from build123d import *

# Parameters (mm, degrees)
F1_DEPTH = 6
F3_DEPTH = 3
F5_DEPTH = 9
F7_DEPTH = 3
F8_R     = 2
F9_R     = 2


with BuildPart() as f1:
    # F0 (on Top) → F1 (new body)
    with BuildSketch(Plane.XY):
        with BuildLine():
            Line((-3, 34.2), (-3, 0))
            ThreePointArc((-3, 0), (-2.1213203436, -2.1213203436), (0, -3))
            Line((0, -3), (34.2, -3))
            Line((34.2, -3), (34.2, 3))
            Line((34.2, 3), (5, 3))
            ThreePointArc((5, 3), (3.5857864376, 3.5857864376), (3, 5))
            Line((3, 5), (3, 34.2))
            Line((3, 34.2), (-3, 34.2))
        make_face()
        with BuildLine():
            Line((1, 32.2), (1, 2))
            ThreePointArc((1, 2), (1.2928932188, 1.2928932188), (2, 1))
            Line((2, 1), (32.2, 1))
            Line((32.2, 1), (32.2, -1))
            Line((32.2, -1), (0, -1))
            ThreePointArc((0, -1), (-0.7071067812, -0.7071067812), (-1, 0))
            Line((-1, 0), (-1, 32.2))
            Line((-1, 32.2), (1, 32.2))
        make_face(mode=Mode.SUBTRACT)
    extrude(amount=F1_DEPTH)

    # F2 (on face) → F3 (join)
    with BuildSketch(Plane.XY.offset(6)):
        with BuildLine():
            Line((3, 34.2), (-3, 34.2))
            Line((-3, 34.2), (-3, 0))
            ThreePointArc((-3, 0), (-2.1213203436, -2.1213203436), (0, -3))
            Line((0, -3), (34.2, -3))
            Line((34.2, -3), (34.2, 3))
            Line((34.2, 3), (5, 3))
            ThreePointArc((5, 3), (3.5857864376, 3.5857864376), (3, 5))
            Line((3, 5), (3, 34.2))
        make_face()
        with BuildLine():
            ThreePointArc((0, -1), (-0.7071067812, -0.7071067812), (-1, 0))
            Line((-1, 0), (-1, 32.2))
            Line((-1, 32.2), (1, 32.2))
            Line((1, 32.2), (1, 2))
            ThreePointArc((1, 2), (1.2928932188, 1.2928932188), (2, 1))
            Line((2, 1), (32.2, 1))
            Line((32.2, 1), (32.2, -1))
            Line((32.2, -1), (0, -1))
        make_face(mode=Mode.SUBTRACT)
        with BuildLine():
            Line((3, 34.2), (-3, 34.2))
            Line((-3, 34.2), (-3, 0))
            ThreePointArc((-3, 0), (-2.1213203436, -2.1213203436), (0, -3))
            Line((0, -3), (34.2, -3))
            Line((34.2, -3), (34.2, 3))
            Line((34.2, 3), (5, 3))
            ThreePointArc((5, 3), (3.5857864376, 3.5857864376), (3, 5))
            Line((3, 5), (3, 34.2))
        make_face()
        with BuildLine():
            Line((-1, 32.2), (-1, 0))
            ThreePointArc((-1, 0), (-0.7071067812, -0.7071067812), (0, -1))
            Line((0, -1), (32.2, -1))
            Line((32.2, -1), (32.2, 1))
            Line((32.2, 1), (2, 1))
            ThreePointArc((2, 1), (1.2928932188, 1.2928932188), (1, 2))
            Line((1, 2), (1, 32.2))
            Line((1, 32.2), (-1, 32.2))
        make_face()
    extrude(amount=F3_DEPTH)

    # F4 (on face) → F5 (join, through all)
    with BuildSketch(Plane(origin=(0, 0, 0), x_dir=(1, 0, 0), z_dir=(0, 0, -1))):
        with BuildLine():
            Line((3, -5), (3, -34.2))
            Line((3, -34.2), (25.1969696197, -34.2))
            Line((25.1969696197, -34.2), (29.6984848098, -29.6984848098))
            Line((29.6984848098, -29.6984848098), (34.2, -25.1969696197))
            Line((34.2, -25.1969696197), (34.2, -3))
            Line((34.2, -3), (5, -3))
            ThreePointArc((5, -3), (3.5857864376, -3.5857864376), (3, -5))
        make_face()
        Polygon((18.9504617358, -29.1327993849), (24.0416305603, -24.0416305603), (29.1327993849, -18.9504617358), (31.9612265096, -21.7788888605), (26.8700576851, -26.8700576851), (21.7788888605, -31.9612265096), align=None, mode=Mode.SUBTRACT)
    extrude(amount=-F5_DEPTH)

    # F6 (on face) → F7 (join)
    with BuildSketch(Plane.XY.offset(9)):
        Polygon((18.9504617358, 29.1327993849), (29.1327993849, 18.9504617358), (31.9612265096, 21.7788888605), (21.7788888605, 31.9612265096), align=None)
    extrude(amount=-F7_DEPTH)

    # F8
    f8_edges = [f1.edges().sort_by_distance(p)[0] for p in [
        (34.2, -3, 4.5),
        (34.2, 25.19697, 4.5),
        (25.19697, 34.2, 4.5),
        (-3, 34.2, 4.5),
    ]]
    fillet(f8_edges, radius=F8_R)

    # F9
    f9_edges = [f1.edges().sort_by_distance(p)[0] for p in [
        (16.1, -3, 9),
        (33.614214, -2.414214, 9),
        (-2.12132, -2.12132, 9),
        (34.2, 11.684271, 9),
        (-3, 16.1, 9),
        (34.047759, 25.133909, 9),
        (-2.414214, 33.614214, 9),
        (29.698485, 29.698485, 9),
        (11.684271, 34.2, 9),
        (25.133909, 34.047759, 9),
    ]]
    fillet(f9_edges, radius=F9_R)


solid = f1.part
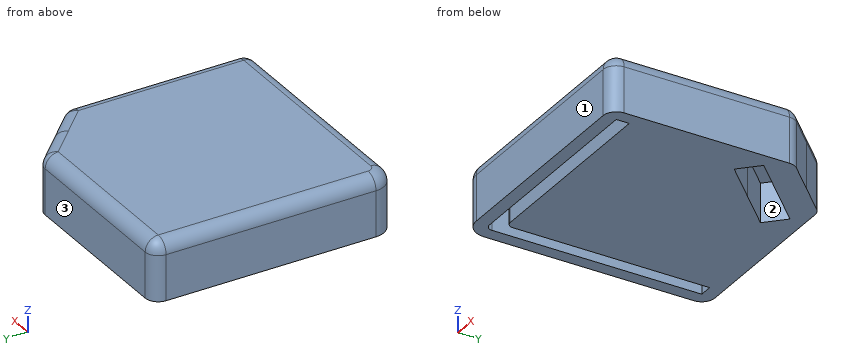
For this review, take the finished solid that the model builds, in its own axes (mm). Face numbers are marked on the shaded views. Round coordinates to 2 decimals unless told otherwise and drop trailing zeros. Loops run counter-clockwise (first coordinate to the right, second up) from the corner with the lowest first, then second, coordinate; pieces in that order, holes last. Notation, with made-up numbers: (58.5, 71) - (102.5, 71) arc R26 cw to (102.5, 103) - close; hole circle Ø6 at (-9, -37). An arc over 180 degrees is marked (long way). One line per item, written item: value. Start each with the question number.
Item 1: For L1, parallel to X at y = 15, z = 5.5; L2, parallel to X at y = 21, z = 2, list the stretches that pass through material, from the lowest coordinate up.
Item 2: Take a section at D-D (x = 20). Give the boundary of the cut face in (y, z), plus the area to 3 significant figures.
Item 3: Clearance check with a flat-ended pin moving along its axis: pin 1 Ø3 at (x, z) = (30, 7) entering from +Y. State where the tip first meets the part, or that it passes through.
Item 4: Take a section at A-A (z = 2.5). Give the boundary of the cut face in (x, y).
Item 5: The part is to be moulded in two halves that separate along Y. For the marked faces 1, 2 and 3, say which applies: +Y half, -Y half, draft (parallel to the pull), parting line (faces both ways), or undercut.
Item 6: Take a section at B-B (x = 10). Give the boundary of the cut face in (y, z), plus the area to 3 significant figures.
Answer below:
1. L1: x = -3 to -1, 1 to 34.2
1. L2: x = -3 to -1, 1 to 27.08, 31.18 to 34.2
2. outline: (-3, 0) - (-1, 0) - (-1, 6) - (1, 6) - (1, 0) - (28.08, 0) - (28.08, 6) - (30.18, 6) - (30.18, 0) - (34.2, 0) - (34.2, 7) arc R2 ccw to (32.2, 9) - (-1, 9) arc R2 ccw to (-3, 7) - close
2. area: 308 mm2
3. pin 1: stops at y = 30.9
4. outline: (-3, 0) arc R3 ccw to (0, -3) - (32.2, -3) arc R2 ccw to (34.2, -1) - (34.2, 24.37) arc R2 ccw to (33.61, 25.78) - (25.78, 33.61) arc R2 ccw to (24.37, 34.2) - (-1, 34.2) arc R2 ccw to (-3, 32.2) - close; hole (-1, 0) arc R1 ccw to (0, -1) - (32.2, -1) - (32.2, 1) - (2, 1) arc R1 cw to (1, 2) - (1, 32.2) - (-1, 32.2) - close; hole (18.95, 29.13) - (29.13, 18.95) - (31.96, 21.78) - (21.78, 31.96) - close
5. face 1: -Y half
5. face 2: undercut
5. face 3: +Y half
6. outline: (-3, 0) - (-1, 0) - (-1, 6) - (1, 6) - (1, 0) - (34.2, 0) - (34.2, 7) arc R2 ccw to (32.2, 9) - (-1, 9) arc R2 ccw to (-3, 7) - close
6. area: 321 mm2
